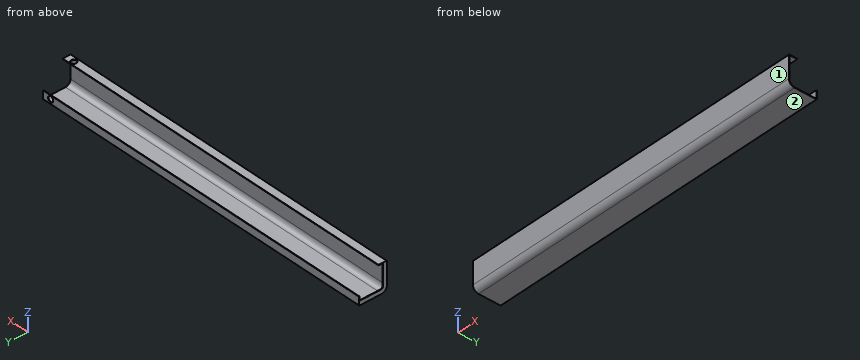
from build123d import *

# Parameters (mm, degrees)
SKETCH_2_W                       = 1250
SKETCH_2_H                       = 100
SM_BASE_FLANGE_1_DEPTH           = 2
SM_EDGE_FLANGE_1_STRIP_W         = 44
SM_EDGE_FLANGE_1_STRIP_H         = 2
SM_EDGE_FLANGE_1_STRIP_CUT_DEPTH = 1250
SM_EDGE_FLANGE_1_DEPTH           = 1250
SM_EDGE_FLANGE_2_STRIP_W         = 9.4732
SM_EDGE_FLANGE_2_STRIP_H         = 2
SM_EDGE_FLANGE_2_STRIP_CUT_DEPTH = 1250
SM_EDGE_FLANGE_2_DEPTH           = 1250
SM_EDGE_FLANGE_3_STRIP_W         = 9.4732
SM_EDGE_FLANGE_3_STRIP_H         = 2
SM_EDGE_FLANGE_3_STRIP_CUT_DEPTH = 1250
SM_EDGE_FLANGE_3_DEPTH           = 1250
SKETCH_16_R                      = 10
CUT_EXTRUDE_1_DEPTH              = 10
SKETCH_17_R                      = 10
CUT_EXTRUDE_2_DEPTH              = 10
EXTRUDE_1_DEPTH                  = 2


# Sheet-metal steps are written as plain solids
with BuildPart() as part:
    # Sketch 2 → 基体-法兰1 (new body)
    with BuildSketch(Plane.XY):
        Rectangle(SKETCH_2_W, SKETCH_2_H)
    extrude(amount=-SM_BASE_FLANGE_1_DEPTH)

    # 边线-法兰1 strip (across the edge) → 边线-法兰1 strip cut (cut)
    with BuildSketch(Plane(origin=(-625, -50, 0), x_dir=(0, 1, 0), z_dir=(1, 0, 0))):
        with Locations((-2, -1)):
            Rectangle(SM_EDGE_FLANGE_1_STRIP_W, SM_EDGE_FLANGE_1_STRIP_H)
    extrude(amount=SM_EDGE_FLANGE_1_STRIP_CUT_DEPTH, mode=Mode.SUBTRACT)

    # 边线-法兰1 section (across the edge) → 边线-法兰1 (add)
    with BuildSketch(Plane(origin=(-625, -50, 0), x_dir=(0, 1, 0), z_dir=(1, 0, 0))):
        with BuildLine():
            Line((0, 18), (0, 98))
            Line((0, 98), (2, 98))
            Line((2, 98), (2, 18))
            ThreePointArc((2, 18), (7.272077939, 5.272077939), (20, 0))
            Line((20, 0), (20, -2))
            ThreePointArc((20, -2), (5.857864376, 3.857864376), (0, 18))
        make_face()
    extrude(amount=SM_EDGE_FLANGE_1_DEPTH)

    # 边线-法兰2 strip (across the edge) → 边线-法兰2 strip cut (cut)
    with BuildSketch(Plane(origin=(625, 50, 0), x_dir=(0, -1, 0), z_dir=(-1, 0, 0))):
        with Locations((-2, -1)):
            Rectangle(SM_EDGE_FLANGE_2_STRIP_W, SM_EDGE_FLANGE_2_STRIP_H)
    extrude(amount=SM_EDGE_FLANGE_2_STRIP_CUT_DEPTH, mode=Mode.SUBTRACT)

    # 边线-法兰2 section (across the edge) → 边线-法兰2 (add)
    with BuildSketch(Plane(origin=(625, 50, 0), x_dir=(0, -1, 0), z_dir=(-1, 0, 0))):
        with BuildLine():
            Line((0, 0.7366), (0, 28))
            Line((0, 28), (2, 28))
            Line((2, 28), (2, 0.7366))
            ThreePointArc((2, 0.7366), (2.215745145, 0.215745145), (2.7366, 0))
            Line((2.7366, 0), (2.7366, -2))
            ThreePointArc((2.7366, -2), (0.801531583, -1.198468417), (0, 0.7366))
        make_face()
    extrude(amount=SM_EDGE_FLANGE_2_DEPTH)

    # 边线-法兰3 strip (across the edge) → 边线-法兰3 strip cut (cut)
    with BuildSketch(Plane(origin=(-625, -48, 98), x_dir=(0, 0, -1), z_dir=(1, 0, 0))):
        with Locations((-2, -1)):
            Rectangle(SM_EDGE_FLANGE_3_STRIP_W, SM_EDGE_FLANGE_3_STRIP_H)
    extrude(amount=SM_EDGE_FLANGE_3_STRIP_CUT_DEPTH, mode=Mode.SUBTRACT)

    # 边线-法兰3 section (across the edge) → 边线-法兰3 (add)
    with BuildSketch(Plane(origin=(-625, -48, 98), x_dir=(0, 0, -1), z_dir=(1, 0, 0))):
        with BuildLine():
            Line((0, 0.7366), (0, 28))
            Line((0, 28), (2, 28))
            Line((2, 28), (2, 0.7366))
            ThreePointArc((2, 0.7366), (2.215745145, 0.215745145), (2.7366, 0))
            Line((2.7366, 0), (2.7366, -2))
            ThreePointArc((2.7366, -2), (0.801531583, -1.198468417), (0, 0.7366))
        make_face()
    extrude(amount=SM_EDGE_FLANGE_3_DEPTH)

    # 草图16 → 切除-拉伸1 (cut)
    with BuildSketch(Plane(origin=(0, 50, 0), x_dir=(1, 0, 0), z_dir=(0, 1, 0))):
        with Locations(Location((595, -15, 0), (0, 0, 270))):
            Circle(SKETCH_16_R)
    extrude(amount=-CUT_EXTRUDE_1_DEPTH, mode=Mode.SUBTRACT)

    # 草图17 → 切除-拉伸2 (cut)
    with BuildSketch(Plane.XY.offset(98)):
        with Locations((595, -33)):
            Circle(SKETCH_17_R)
    extrude(amount=-CUT_EXTRUDE_2_DEPTH, mode=Mode.SUBTRACT)

    # 草图30 → 凸台-拉伸1 (add)
    with BuildSketch(Plane.ZY.offset(625)):
        with BuildLine():
            Line((13, 50), (0.7366, 50))
            ThreePointArc((0.7366, 50), (-1.198468417, 49.198468417), (-2, 47.2634))
            Line((-2, 47.2634), (-2, -30))
            ThreePointArc((-2, -30), (3.857864376, -44.142135624), (18, -50))
            Line((18, -50), (95.2634, -50))
            ThreePointArc((95.2634, -50), (97.198468417, -49.198468417), (98, -47.2634))
            Line((98, -47.2634), (98, -35))
            Line((98, -35), (18, -35))
            ThreePointArc((18, -35), (14.464466094, -33.535533906), (13, -30))
            Line((13, -30), (13, 50))
        make_face()
    extrude(amount=-EXTRUDE_1_DEPTH)


solid = part.part
Geometry: final body of the model. Coordinates: model frame, mm. Face numbers are marked on the shaded views. Give positions to 0.01 mm unless a question says otherwise; leave off trailing zeros. Order: outer loops, then holes, each group sorted by start corner. A loop starts at its lowest first (then second) coordinate and runs counter-clockwise, first axis right, second up. Notation, with made-up numbers: (89.5, 18.25) -> (130.5, 18.25) arc R26 ccw to (130.5, 49.25) -> close; hole circle Ø5 at (-27.75, 30). An arc over 180 degrees is marked (long way). Answer as a JSON object with one key per item and string values.
Q1. First-contact query: pin 1 (0.6 mm diameter, centred on x = -624, z = 66, fed in from +Y); pin 2 (1 mm diameter, centred on x = -623.5, y = 15.5, fed in from +Z); pin 3 (5 mm diameter, centred on x = -490, y = 5, fed in from +Z). Flat tips, straight axial feed; report the tip coordinate or a pass-through.
Entries:
{"pin 1": "stops at y = -35", "pin 2": "stops at z = 13", "pin 3": "stops at z = 0"}
Q2. Section A-A (x = 20). Output: boundary loops of the cut face in (y, z).
Entries:
{"outline": "(-50, 18) arc R20 ccw to (-30, -2) -> (47.26, -2) arc R2.74 ccw to (50, 0.74) -> (50, 28) -> (48, 28) -> (48, 0.74) arc R0.74 cw to (47.26, 0) -> (-30, 0) arc R18 cw to (-48, 18) -> (-48, 95.26) arc R0.74 cw to (-47.26, 96) -> (-20, 96) -> (-20, 98) -> (-47.26, 98) arc R2.74 ccw to (-50, 95.26) -> close"}
Q3. Section C-C (y = 1). Output: boundary loops of the cut face in (x, z).
Entries:
{"outline": "(-625, -2) -> (625, -2) -> (625, 0) -> (-623, 0) -> (-623, 13) -> (-625, 13) -> close"}
Q4. Section B-B (z = 61). Output: boundary loops of the cut face in (x, y).
Entries:
{"outline": "(-625, -50) -> (625, -50) -> (625, -48) -> (-623, -48) -> (-623, -35) -> (-625, -35) -> close"}
Q5. Material intervals for probe 1 along Y at (x, z) = (3.5, 20); probe 2 along Z at (x, y) = (-409.5, -26); probe 3 along Z at (x, y) = (530.5, 35.5), sorted ascending.
Entries:
{"probe 1": "y = -50 to -48, 48 to 50", "probe 2": "z = -2 to 0, 96 to 98", "probe 3": "z = -2 to 0"}
Q6. Draft query along Z for the marked faces 1 and 2. Return one class per face: released by +Z, released by -Z, zero draft, split by the parting line, or undercut.
Entries:
{"face 1": "zero draft", "face 2": "released by -Z"}
